Could you check a few things on this drawing? It's one solid part, dimensions in mm from its lowest x, y, z. A direction names the side the tool comes from. Round coordinates to 2 decimals unless told otherwise and drop trailing zeros. Write each loop counter-clockwise with the first axis right and the second up, starting at its lowest first coordinate (ties: lowest second). Pieces come first, ordered by that corner, then holes. Notation, with made-up numbers: (38, 79.5) -> (57, 79.5) arc R11 ccw to (57, 95.5) -> close; hole circle Ø11 at (3.5, -12). An arc over 180 degrees is marked (long way). Answer in a Markdown table with one row per item. Add a question column.
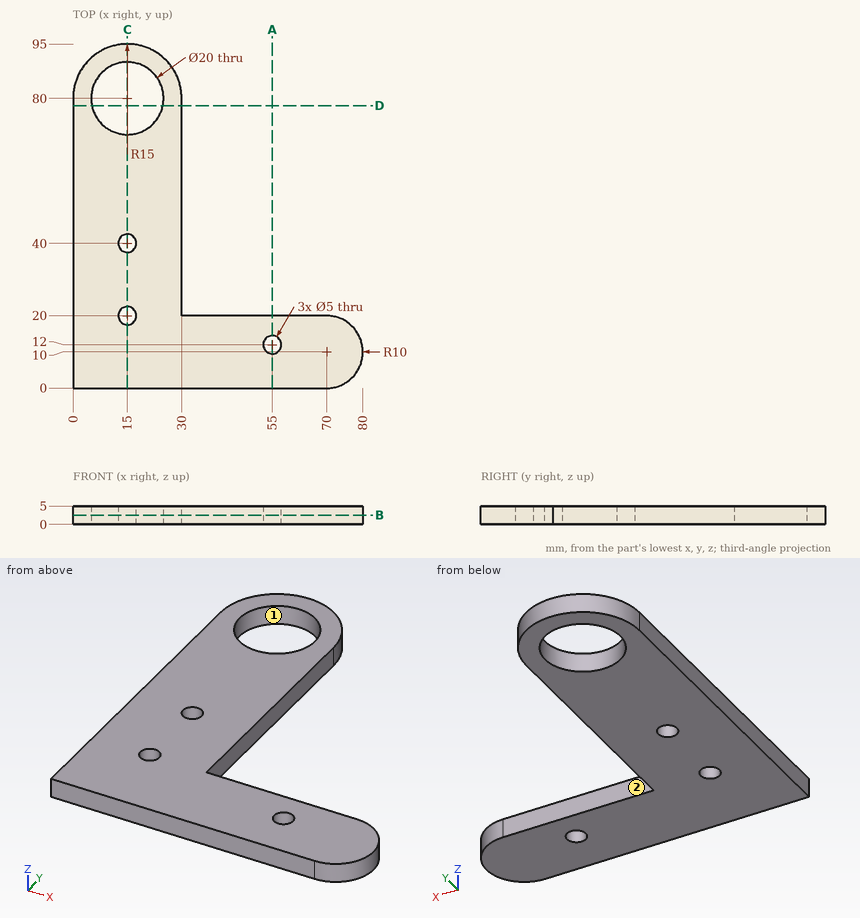
(1) Suppose I cut it at C-C, the plane x = 15. Please give me the cut outline in (y, z).
(2) Suppose I cut it at A-A, the plane x = 55. Please give me the cut outline in (y, z), then the cut area to 3 significant figures.
(3) On a 3-axis mill with a long thin cutter (end or side, diameter ignored), from which of +Z, -Z, +X, -X, +Y, -Y can I reach the whole of each face in a straight line? I mean the marked faces 1 and 2. Say none if no direction works.
(4) Suppose I cut it at B-B, the plane z = 2.5. Please give me the cut outline in (x, y), then the cut area to 3 significant figures.
(5) For P1, Ø1, axis at y = 55, z = 2.5, coming from the +X side; P2, Ø1.5, axis at x = 41, z = 2.5, coming from the +Y side, each with a flat end and sliding along its axis, tell me the tip position at first contact or that it passes through.
(6) Suppose I cut it at D-D, the plane y = 78. Please give me the cut outline in (x, z).
(7) I need wall thicknesses on L1, parallel to Y at x = 15, z = 1.4; L2, parallel to Y at x = 55, z = 1.25; L3, parallel to X at y = 58, z = 2.45. Which ranges of each line are inside material? Lowest first, please.
Response:
| question | item | result |
|---|---|---|
| 1 | outline | (0, 0) -> (17.5, 0) -> (17.5, 5) -> (0, 5) -> close; (22.5, 0) -> (37.5, 0) -> (37.5, 5) -> (22.5, 5) -> close; (42.5, 0) -> (70, 0) -> (70, 5) -> (42.5, 5) -> close; (90, 0) -> (95, 0) -> (95, 5) -> (90, 5) -> close |
| 2 | outline | (0, 0) -> (9.5, 0) -> (9.5, 5) -> (0, 5) -> close; (14.5, 0) -> (20, 0) -> (20, 5) -> (14.5, 5) -> close |
| 2 | area | 75.0 mm² |
| 3 | face 1 | +Z, -Z |
| 3 | face 2 | +Z, -Z, +X, +Y |
| 4 | outline | (0, 0) -> (70, 0) arc R10 ccw to (70, 20) -> (30, 20) -> (30, 80) arc R15 ccw to (0, 80) -> close; hole circle Ø20 at (15, 80); hole circle Ø5 at (15, 20); hole circle Ø5 at (15, 40); hole circle Ø5 at (55, 12) |
| 4 | area | 3,340 mm² |
| 5 | P1 | x = 30 |
| 5 | P2 | y = 20 |
| 6 | outline | (0, 0) -> (5.2, 0) -> (5.2, 5) -> (0, 5) -> close; (24.8, 0) -> (30, 0) -> (30, 5) -> (24.8, 5) -> close |
| 7 | L1 | 0 to 17.5, 22.5 to 37.5, 42.5 to 70, 90 to 95 |
| 7 | L2 | 0 to 9.5, 14.5 to 20 |
| 7 | L3 | 0 to 30 |
